Read the model definition and answer for the solid it produces. Units are mm, in the model's axes. Give positions to 0.01 mm unless a question says otherwise; leave off trailing zeros. Loops run counter-clockwise (first coordinate to the right, second up) from the corner with the lowest first, then second, coordinate; pieces in that order, holes last. Notation, with made-up numbers: (-12, 34.25) - (46, 34.25) arc R25 cw to (46, 71.25) - close; hole circle Ø3 at (20.25, -36.5). An arc over 180 degrees is marked (long way). Write item = value, one per line.
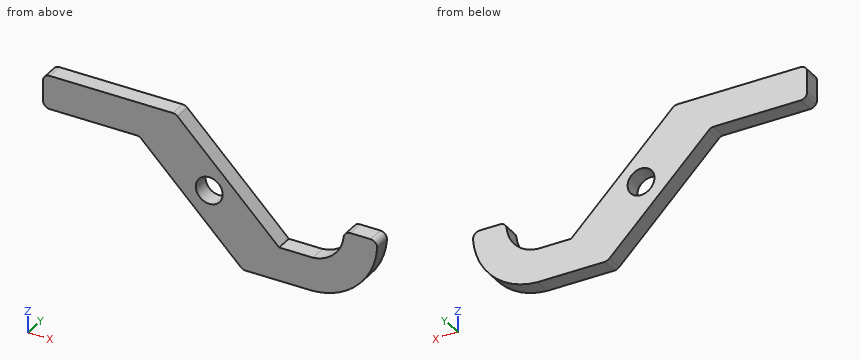
```python
from build123d import *

# Parameters (mm, degrees)
SKETCH1_R           = 5.08
BOSS_EXTRUDE1_DEPTH = 6.35


with BuildPart() as part:
    # Sketch1 → Boss-Extrude1 (new body)
    with BuildSketch(Plane(origin=(0, 0, 0), x_dir=(1, 0, 0), z_dir=(0, 1, 0))):
        with BuildLine():
            Line((-11.956051224, 0.073941191), (26.403889176, 38.433881591))
            Line((26.403889176, 38.433881591), (39.103889176, 38.433881591))
            ThreePointArc((39.103889176, 38.433881591), (47.009448875, 34.839896868), (50.775072277, 27.014637718))
            ThreePointArc((50.775072277, 27.014637718), (51.59882499, 25.385821387), (53.302203848, 24.729992415))
            Line((53.302203848, 24.729992415), (60.928206609, 24.729992415))
            ThreePointArc((60.928206609, 24.729992415), (62.783570301, 25.53528046), (63.462475569, 27.440523463))
            ThreePointArc((63.462475569, 27.440523463), (55.823997921, 43.955508609), (39.103889176, 51.133881591))
            Line((39.103889176, 51.133881591), (13.752102448, 51.133881591))
            ThreePointArc((13.752102448, 51.133881591), (12.78008653, 50.940535604), (11.956051224, 50.389932815))
            Line((11.956051224, 50.389932815), (-25.6599404, 12.773941191))
            ThreePointArc((-25.6599404, 12.773941191), (-26.483975706, 12.223338403), (-27.455991624, 12.029992415))
            Line((-27.455991624, 12.029992415), (-60.230604195, 12.029992415))
            ThreePointArc((-60.230604195, 12.029992415), (-62.026655419, 11.28604364), (-62.770604195, 9.489992415))
            Line((-62.770604195, 9.489992415), (-62.770604195, 1.869992415))
            ThreePointArc((-62.770604195, 1.869992415), (-62.026655419, 0.073941191), (-60.230604195, -0.670007585))
            Line((-60.230604195, -0.670007585), (-13.752102448, -0.670007585))
            ThreePointArc((-13.752102448, -0.670007585), (-12.78008653, -0.476661597), (-11.956051224, 0.073941191))
        make_face()
        with Locations(Location((0, 24.729992415, 0), (0, 0, 270))):
            Circle(SKETCH1_R, mode=Mode.SUBTRACT)
    extrude(amount=BOSS_EXTRUDE1_DEPTH)


solid = part.part
```
1) A cutting plane is placed at A-A on x = 0. Determine the outline of the cut face in (y, z), then the cut area to 3 significant figures.
Output:
outline = (0, -38.43) - (6.35, -38.43) - (6.35, -29.81) - (0, -29.81) - close; (0, -19.65) - (6.35, -19.65) - (6.35, -12.03) - (0, -12.03) - close
area = 103 mm²
2) Each of these flat-tipped pins is pushed along its axis until it touches: P1, Ø2, axis at y = 3, z = -17, coming from the -X side; P2, Ø1.9, axis at x = -37.5, y = 2.5, coming from the -Z side; P3, Ø6, axis at x = 0, z = -24.73, coming from the -Y side; P4, Ø3, axis at y = 2, z = -31.5, coming from the +X side. Where does it stop, or does it pass through?
Output:
P1 = -22.43
P2 = -12.03
P3 = through
P4 = 63.16
3) A cutting plane is placed at B-B on y = 2.5. Determine the outline of the cut face in (x, z), then the cut area to 3 significant figures.
Output:
outline = (-62.77, -9.49) arc R2.54 ccw to (-60.23, -12.03) - (-27.46, -12.03) arc R2.54 cw to (-25.66, -12.77) - (11.96, -50.39) arc R2.54 ccw to (13.75, -51.13) - (39.1, -51.13) arc R25.42 ccw to (63.46, -27.44) arc R2.54 ccw to (60.93, -24.73) - (53.3, -24.73) arc R2.54 ccw to (50.78, -27.01) arc R12.74 cw to (39.1, -38.43) - (26.4, -38.43) - (-11.96, -0.07) arc R2.54 ccw to (-13.75, 0.67) - (-60.23, 0.67) arc R2.54 ccw to (-62.77, -1.87) - close; hole circle Ø10.16 at (0, -24.73)
area = 2,120 mm²
4) A cutting plane is placed at D-D on z = -5. Determine the outline of the cut face in (x, y).
Output:
outline = (-62.77, 0) - (-7.03, 0) - (-7.03, 6.35) - (-62.77, 6.35) - close
5) A cutting plane is placed at C-C on z = -36. Determine the outline of the cut face in (x, y), then the cut area to 3 significant figures.
Output:
outline = (-2.43, 0) - (23.97, 0) - (23.97, 6.35) - (-2.43, 6.35) - close; (45.64, 0) - (61.35, 0) - (61.35, 6.35) - (45.64, 6.35) - close
area = 267 mm²
6) Find the intervals of material crossed by probe 1 along Z at (x, y) = (-46, 2.5); probe 2 along Z at (x, y) = (29, 3); probe 3 along X at (y, z) = (6, -30.5), in increasing order.
Output:
probe_1 = -12.03 to 0.67
probe_2 = -51.13 to -38.43
probe_3 = -7.93 to 18.47, 49.91 to 63.07
